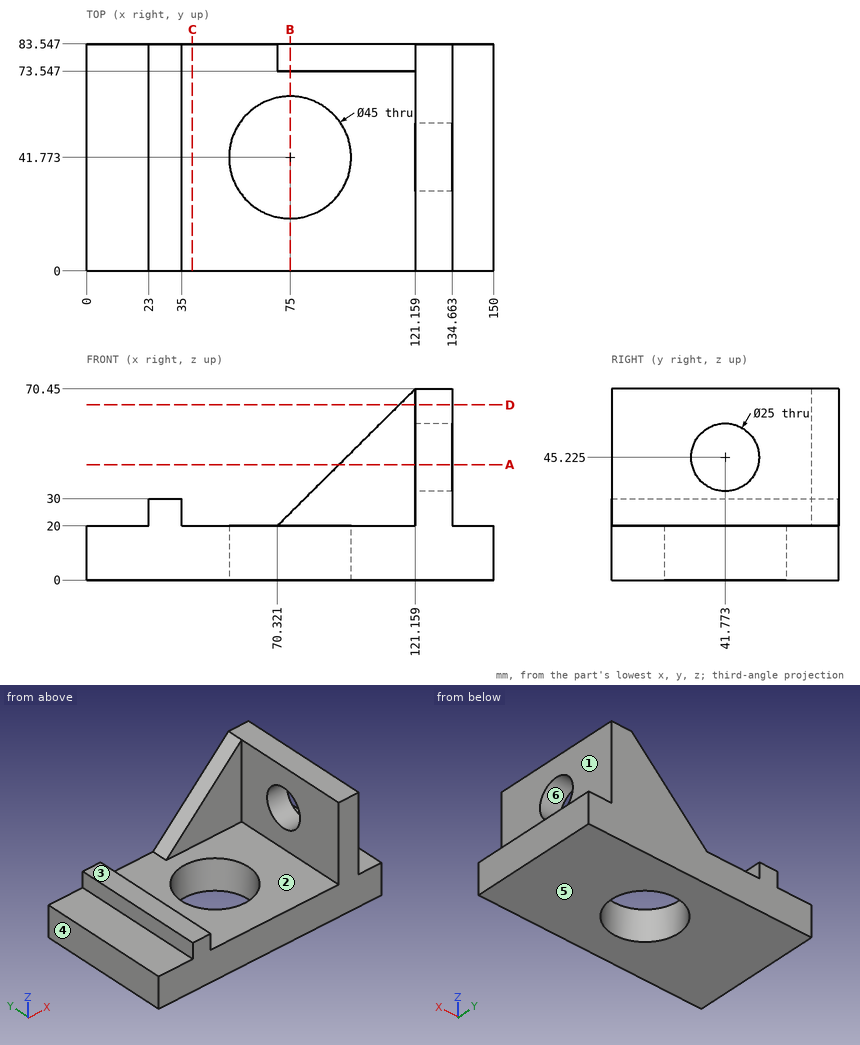
Design review of the part shown in the three views and the two pictorial views. Dimensions are in mm from the part's minimum x, y and z. A direction names the side the tool comes from. Round coordinates to 2 decimals unless told otherwise and drop trailing zeros. Loops run counter-clockwise (first coordinate to the right, second up) from the corner with the lowest first, then second, coordinate; pieces in that order, holes last. Notation, with made-up numbers: (83, -25.5) -> (130, -25.5) arc R17 cw to (130, -16.5) -> close; hole circle Ø2 at (-33, 89.5). An arc over 180 degrees is marked (long way). Use one line per item in the form item = value. Start each with the question number.
Q1. We need section A-A on z = 42.5. Give the boundary of the cut face in (x, y) (1 decimal).
Q2. Draft analysis for pull direction Z (two halves, no side actions). For the marked faces 4, 5 and 6, state which applies: +Z half, -Z half, draft (parallel to the pull), parting line (faces both ways), or undercut.
Q3. For pin 1 Ø4.5 at (x, y) = (145.5, 46) entering from +Z; pin 2 Ø25 at (y, z) = (28.5, 49) entering from -X; pin 3 Ø2 at (y, z) = (59, 58) entering from +X; pin 4 Ø3 at (x, y) = (34.5, 75) entering from -Z, all flat-tipped, find the tip position at first contact; note any pin that passes through.
Q4. We need section B-B on x = 75. Give the boundary of the cut face in (y, z).
Q5. We need section C-C on x = 39. Give the boundary of the cut face in (y, z), then the cut area to 3 significant figures.
Q6. Wall thickness on line 1 along X through (y, z) = (35, 26); line 2 along Y through (x, z) = (75, 8); line 3 along X through (y, z) = (55.5, 43.5): over which ranges is each line inside the solid? List them lowest first. Write a range as [from, to].
Q7. We need section D-D on z = 64.5. Give the boundary of the cut face in (x, y), then the cut area to 3 significant figures.
Q8. Machinability: for the marked faces 1, 2 and 3, which of the approach directions +Z, -Z, +X, -X, +Y, -Y give a long, thin tool a straight path to every point of the face, cutting with its end or side? Answer none if there is none.
Calculated:
q1.outline = (93, 73.5) -> (121.2, 73.5) -> (121.2, 54) -> (134.7, 54) -> (134.7, 83.5) -> (93, 83.5) -> close; (121.2, 0) -> (134.7, 0) -> (134.7, 29.6) -> (121.2, 29.6) -> close
q2.face_4 = draft
q2.face_5 = -Z half
q2.face_6 = undercut
q3.pin_1 = 20
q3.pin_2 = 121.16
q3.pin_3 = 134.66
q3.pin_4 = 0
q4.outline = (0, 0) -> (19.27, 0) -> (19.27, 20) -> (0, 20) -> close; (64.27, 0) -> (83.55, 0) -> (83.55, 24.64) -> (73.55, 24.64) -> (73.55, 20) -> (64.27, 20) -> close
q5.outline = (0, 0) -> (83.55, 0) -> (83.55, 20) -> (0, 20) -> close
q5.area = 1,670 mm²
q6.line_1 = [23, 35], [121.16, 134.66]
q6.line_2 = [0, 19.27], [64.27, 83.55]
q6.line_3 = [121.16, 134.66]
q7.outline = (115.16, 73.55) -> (121.16, 73.55) -> (121.16, 0) -> (134.66, 0) -> (134.66, 83.55) -> (115.16, 83.55) -> close
q7.area = 1,190 mm²
q8.face_1 = +Z, +X, +Y, -Y
q8.face_2 = +Z, -Y
q8.face_3 = +Z, -X, +Y, -Y
